Source: CAD feature listing. Evaluate the final solid. Frame: model axes, mm. Face numbers are marked on the shaded views. A direction names the side the tool comes from. Coordinates: 2 decimals unless noted, no trailing zeros. Order: outer loops, then holes, each group sorted by start corner. A loop starts at its lowest first (then second) coordinate and runs counter-clockwise, first axis right, second up.
```python
from build123d import *

# Parameters (mm, degrees)
F1_DEPTH = 20.32


with BuildPart() as f1:
    # F0 (on Front) → F1 (new body)
    with BuildSketch(Plane.XZ):
        with BuildLine():
            Line((2.483238, 13.186188), (-3.866762, 13.186188))
            Line((-3.866762, 13.186188), (-16.566762, 13.186188))
            Line((-16.566762, 13.186188), (-16.566762, 12.186188))
            Line((-16.566762, 12.186188), (-3.866762, 12.186188))
            Line((-3.866762, 12.186188), (-3.866762, 11.186188))
            Line((-3.866762, 11.186188), (0.483238, 11.186188))
            ThreePointArc((0.483238, 11.186188), (13.953622, 5.606572), (19.533238, -7.863812))
            Line((19.533238, -7.863812), (19.533238, -12.213812))
            Line((19.533238, -12.213812), (20.533238, -12.213812))
            Line((20.533238, -12.213812), (20.533238, -24.913812))
            Line((20.533238, -24.913812), (21.533238, -24.913812))
            Line((21.533238, -24.913812), (21.533238, -12.213812))
            Line((21.533238, -12.213812), (21.533238, -5.863812))
            ThreePointArc((21.533238, -5.863812), (15.953622, 7.606572), (2.483238, 13.186188))
        make_face()
    extrude(amount=F1_DEPTH)


solid = f1.part
```
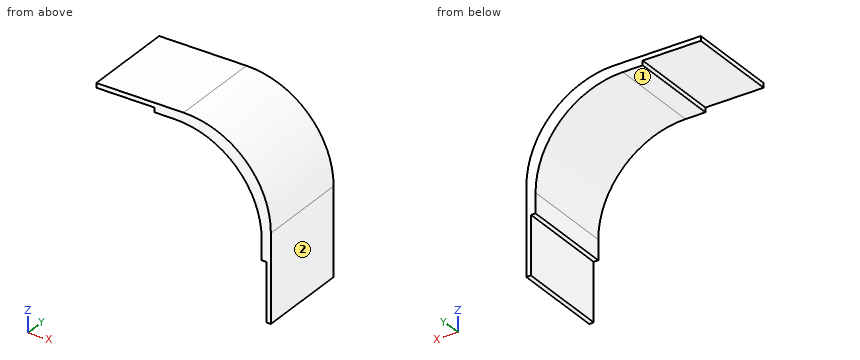
Q1. Set-up query: the marked faces 1 and 2. Return all of +Z, -Z, +X, -X, +Y, -Y with unobstructed straight access to the full face (end or side cutting, diameter ignored); none if empty.
Solutions:
face 1: -Z, -X, +Y, -Y
face 2: +Z, -Z, +X, +Y, -Y
Q2. Pin query (flat end, axial travel): P1, Ø1.5, axis at y = -12.5, z = 6.5, coming from the +X side; P2, Ø0.8, axis at y = -6, z = 11.5, coming from the -X side; P3, Ø1.5, axis at y = -5.5, z = -6, coming from the -X side; P4, Ø3, axis at x = 6.5, z = 8, coming from the +Y side. Return the tip coordinate at first contact, or that it passes through.
Solutions:
P1: stops at x = 17.58
P2: stops at x = -3.87
P3: stops at x = 19.35
P4: passes through
Q3. Section query C-C on z = -4. Output: boundary loops of the cut face in (x, y), plus the area to 3 significant figures.
Solutions:
outline: (19.14, -20.32) - (21.44, -20.32) - (21.44, 0) - (19.14, 0) - close
area: 46.8 mm2
Q4. Section query B-B on x = -2.5. Output: boundary loops of the cut face in (y, z), plus the area to 3 significant figures.
Solutions:
outline: (-20.32, 11.19) - (0, 11.19) - (0, 13.19) - (-20.32, 13.19) - close
area: 40.6 mm2
Q5. Section query A-A on y = -16. Output: boundary loops of the cut face in (x, z), plus the area to 3 significant figures.
Solutions:
outline: (-16.57, 12.19) - (-3.87, 12.19) - (-3.87, 11.19) - (0.48, 11.19) arc R19.05 cw to (19.53, -7.86) - (19.53, -12.21) - (20.53, -12.21) - (20.53, -24.91) - (21.53, -24.91) - (21.53, -5.86) arc R19.05 ccw to (2.48, 13.19) - (-16.57, 13.19) - close
area: 123 mm2
Q6. Material intervals for line 1 along Z through (x, y) = (-2.5, -1.5); line 2 along Z through (x, y) = (-12, -18.75); line 3 along X through (y, z) = (-7.5, -20.5), sorted ascending.
Solutions:
line 1: z = 11.19 to 13.19
line 2: z = 12.19 to 13.19
line 3: x = 20.53 to 21.53
